Input: part model. Units: mm. Frame: model coordinates. Face numbers are marked on the shaded views. A direction names the side the tool comes from. Give positions to 0.01 mm unless a question says otherwise; leave off trailing zeros. Loops run counter-clockwise (first coordinate to the right, second up) from the corner with the lowest first, then second, coordinate; pieces in that order, holes last. Notation, with made-up numbers: M 86.25,44 L 116.25,44 A12 cw 116.25,52 Z; hole C 55.5,34 d1. An arc over 180 degrees is marked long. One line per item, written item: value. Start each with the question number.
(1) Pin query (flat end, axial travel): P1, Ø5, axis at x = -24, z = 5, coming from the -Y side; P2, Ø11.5, axis at x = 9, z = 12.5, coming from the +Y side; P3, Ø8, axis at y = -27, z = 7.5, coming from the +X side. Return the tip coordinate at first contact, or that it passes through.
(2) Section B-B on x = -23.5. Output: boundary loops of the cut face in (y, z), plus the area to 3 significant figures.
(3) Ray query, line 1 along Y through (x, z) = (-15.5, 20.75); line 2 along X through (y, z) = (-26, 11); line 3 along Y through (x, z) = (-31.5, 4). Return the intervals inside material, ascending. Write a range as from..to.
(4) Pull-direction query (X, two-part tool) for the marked faces 1, 2, 3 and 4; classes: released by +X, released by -X, zero draft, split by the parting line, or undercut.
(5) Section A-A on z = 10.5. Output: boundary loops of the cut face in (x, y), plus the area to 3 significant figures.
(6) Section C-C on y = 2. Output: boundary loops of the cut face in (x, z), plus the area to 3 significant figures.
(7) Access query for the marked faces 5, 6 and 7. Directions: +Z, -Z, +X, -X, +Y, -Y. A direction counts if a zero-diameter tool reaches every point of the face in a straight line with its end or side. Return the directions, or none.
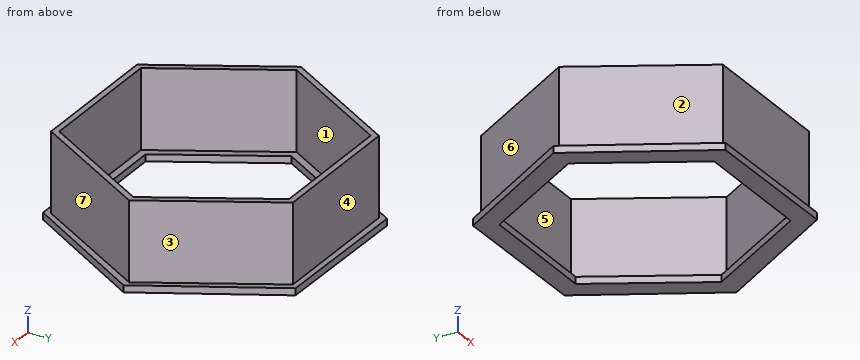
```python
from build123d import *

# Parameters (mm, degrees)
F1_DEPTH = 25
F3_DEPTH = 2
F5_DEPTH = 15.1


with BuildPart() as f1:
    # F0 (on Top) → F1 (new body)
    with BuildSketch(Plane.XY):
        Polygon((20.207259, -35), (40.414519, 0), (20.207259, 35), (-20.207259, 35), (-40.414519, 0), (-20.207259, -35), align=None)
        Polygon((19.196896, 33.25), (38.393793, 0), (19.196896, -33.25), (-19.196896, -33.25), (-38.393793, 0), (-19.196896, 33.25), align=None, mode=Mode.SUBTRACT)
    extrude(amount=F1_DEPTH)

    # F2 (on Top) → F3 (join)
    with BuildSketch(Plane.XY):
        Polygon((20.888331, -36.919732), (42.417591, -0.370041), (21.52926, 36.549691), (-20.888331, 36.919732), (-42.417591, 0.370041), (-21.52926, -36.549691), align=None)
    extrude(amount=F3_DEPTH)

    # F4 (on Top) → F5 (cut)
    with BuildSketch(Plane.XY):
        Polygon((17.955634, -31.100071), (35.911268, 0), (17.955634, 31.100071), (-17.955634, 31.100071), (-35.911268, 0), (-17.955634, -31.100071), align=None)
    extrude(amount=F5_DEPTH, mode=Mode.SUBTRACT)


solid = f1.part
```
Output values:
1. P1: stops at y = -32.76
1. P2: stops at y = 35
1. P3: stops at x = 27.14
2. outline: M -33.07,0 L -21.5,0 L -21.5,2 L -25.8,2 L -25.8,25 L -29.3,25 L -29.3,2 L -33.07,2 Z; M 21.5,0 L 32.49,0 L 32.49,2 L 29.3,2 L 29.3,25 L 25.8,25 L 25.8,2 L 21.5,2 Z
2. area: 206 mm²
3. line 1: y = -35..-33.25, 33.25..35
3. line 2: x = -25.4..-23.38, 23.38..25.4
3. line 3: y = -15.44..-11.94, 11.94..15.44
4. face 1: undercut
4. face 2: released by -X
4. face 3: released by +X
4. face 4: zero draft
5. outline: M -40.41,0 L -20.21,-35 L 20.21,-35 L 40.41,0 L 20.21,35 L -20.21,35 Z; hole M -38.39,0 L -19.2,-33.25 L 19.2,-33.25 L 38.39,0 L 19.2,33.25 L -19.2,33.25 Z
5. area: 414 mm²
6. outline: M -41.46,0 L -34.76,0 L -34.76,2 L -37.24,2 L -37.24,25 L -39.26,25 L -39.26,2 L -41.46,2 Z; M 34.76,0 L 41.08,0 L 41.08,2 L 39.26,2 L 39.26,25 L 37.24,25 L 37.24,2 L 34.76,2 Z
6. area: 119 mm²
7. face 5: +Z
7. face 6: +Z, -X, +Y
7. face 7: +Z, +X, -Y
